Autodesk Inventor part; units mm, degrees
ref_plane "YZ Plane" through (0, 0, 0) normal (1, 0, 0) x (0, 1, 0)
ref_plane "XZ Plane" through (0, 0, 0) normal (0, 1, 0) x (-1, 0, 0)
ref_plane "XY Plane" through (0, 0, 0) normal (0, 0, 1) x (1, 0, 0)
sketch "Sketch1" plane through (0, 0, 0) normal (0, 1, 0) x (-1, 0, 0)
  line L0 (-25, 25) -> (25, 25)
  line L1 (25, 25) -> (25, -25)
  line L2 (25, -25) -> (-25, -25)
  line L3 (-25, -25) -> (-25, 25)
  line L4 (-25, 25) -> (25, -25) construction
  line L5 (25, 25) -> (-25, -25) construction
  line L6 (25, 0) -> (-25, 0)
  circle A0 centre (12.5, 15.25) radius 1.75
  line L7 (-25, 12.5) -> (0, 12.5)
  line L8 (-12.5, 12.5) -> (-12.5, 0)
  circle A1 centre (-12.5, 6.25) radius 1.75
  line L9 (25, -25) -> (-25, 25) construction
  circle A2 centre (12.5, -15.25) radius 1.75
  circle A3 centre (-12.5, -6.25) radius 1.75
  line L10 (0, 32.5) -> (50, 32.5)
  line L11 (50, 32.5) -> (50, -32.5)
  line L12 (50, -32.5) -> (0, -32.5)
  line L13 (0, -32.5) -> (0, 32.5)
  line L14 (0, 32.5) -> (50, -32.5) construction
  line L15 (50, 32.5) -> (0, -32.5) construction
  line L16 (50, -32.5) -> (29.5652, -32.5)
  line L17 (29.5652, -32.5) -> (29.5652, 32.5)
  line L18 (29.5652, 32.5) -> (50, 32.5)
  line L19 (0, 32.5205) -> (0, -32.5)
  circle A4 centre (12.5, -15.25) radius 15
  line L20 (29.5652, -32.5) -> (39.5652, -32.5)
  line L21 (39.5652, -32.5) -> (39.5652, 32.5)
  line L22 (39.5652, 32.5) -> (29.5652, 32.5)
  line L23 (29.5652, 32.5) -> (29.5652, -32.5)
  line L24 (12.5, -15.25) -> (12.5, 0)
  line L25 (-12.5, -6.25) -> (12.5, -6.25)
  circle A5 centre (-4, 0) radius 5
  circle A6 centre (-4, 0) radius 1.75
  line L26 (0, 0) -> (-4, 0)
  line L27 (29.5652, -32.5) -> (29.5652, -27.5)
  line L28 (29.5652, -27.5) -> (34.5652, -27.5)
  line L29 (34.5652, -27.5) -> (34.5652, 27.5)
  line L30 (34.5652, 27.5) -> (29.5652, 27.5)
  line L31 (29.5652, 27.5) -> (29.5652, -27.5)
  point P0 (0, -12.5)
  point P1 (-12.5, -12.5)
  point P2 (0, 25)
  point P3 (0, -25)
  point P4 (0, 25)
  point P5 (0, -25)
  point P6 (0, 32.5)
  point P7 (0, 32.5)
  point P8 (0, -23.5416)
  point P9 (1.101, -25)
  point P10 (25, -23.5416)
  point P11 (23.899, -25)
  point P12 (39.5652, 32.5)
  point P13 (0, 0)
  dimension "d0" = 50
  dimension "d1" = 50
  dimension "d5" = 3.5
  dimension "d7" = 3.5
  dimension "d11" = 15.25
  dimension "d12" = 50
  dimension "d13" = 65
  dimension "d19" = 30
  dimension "d21" = 10
  dimension "d27" = 7.5
  dimension "d28" = 7.5
  dimension "d31" = 9
  dimension "d32" = 25
  dimension "d57" = 10
  dimension "d58" = 3.5
  dimension "d59" = 4
  dimension "d60" = 5
  dimension "d61" = 55
extrude "Extrusion3" add sketch "Sketch1" along normal blind 5 contours L0 L13 L7 L3 | L13 L10 L17 L12 L2 A4 L1 L0 | L0 L1 L6 A5 L13 | L7 L8 A1 L6 L3 | L13 A5 L6 L8 A1 L7 | L6 A5 L13 A4 L2 L3 | L1 A4 L24 L6 | A5 L6 L13 | L13 L6 A6 A5 | A4 L1 | L1 A4 L2 L13 L25 L24 | L24 A4 L25 L13 A5 L6 | L13 A5 L6 A6 | L6 A5 L13 | L30 L29 L28 L17 | L13 A4 L2 | L1 L2 A4 | L24 L25 A4 | L2 A4 | A4 L13 | A4 L13 L25 | A0
fillet "Fillet5" radius 12 2 edges at (0, 2.5, 32.5) (0, 2.5, -32.5)
fillet "Fillet6" radius 12 2 edges at (0, 2.5, 25) (0, 2.5, -25)
fillet "Fillet7" radius 18.5 2 edges at (25, 2.5, 25) (25, 2.5, -25)
sketch "Sketch5" plane through (0, 5, 0) normal (0, 1, 0) x (1, 0, 0)
  circle A0 centre (-12.5, 15.25) radius 1.75
  circle A1 centre (-12.5, -15.25) radius 1.5
  circle A2 centre (-12.5, -15.25) radius 5
  circle A3 centre (4, 0) radius 1.75
  circle A4 centre (4, 0) radius 3
  circle A5 centre (12.5, 6.25) radius 1.75
  circle A6 centre (12.5, 6.25) radius 3
  circle A7 centre (12.5, -6.25) radius 1.75
  circle A8 centre (12.5, -6.25) radius 3
  circle A9 centre (-12.5, 15.25) radius 3
  point P0 (0, 0)
  dimension "d63" = 6
  dimension "d64" = 6
  dimension "d65" = 6
  dimension "d71" = 10
  dimension "d75" = 6
extrude "Extrusion8" cut sketch "Sketch5" against normal blind 2 contours A3 | A4 | A5 | A6 | A7 | A8
fillet "Fillet9" radius 2 11 edges at (6.4021, 5, 25) (1.5607, 5, 25.9773) (-6.3809, 5, 31.5227) (-20.3448, 5, 32.5) (25, 5, 0) (19.5815, 5, -19.5815) (6.4021, 5, -25) (1.5607, 5, -25.9773) (-6.3809, 5, -31.5227) (-20.3448, 5, -32.5) (19.5815, 5, 19.5815)
extrude "Extrusion9" cut sketch "Sketch5" against normal through all contours A1 | A2
sketch "Sketch6" plane through (0, 0, 0) normal (0, -1, 0) x (1, 0, 0)
  circle A0 centre (-12.5, -15.25) radius 1.75
  circle A1 centre (-12.5, -15.25) radius 5
  point P0 (0, 0)
  dimension "d72" = 10
extrude "Extrusion10" cut sketch "Sketch6" against normal blind 2
extrude "Extrusion11" cut sketch "Sketch5" against normal blind 2 contours A0 | A9
sketch "Sketch7" plane through (0, 0, 0) normal (0, -1, 0) x (1, 0, 0)
  circle A0 centre (-12.5, 15.25) radius 5
  circle A1 centre (-12.5, -15.25) radius 5
  point P0 (0, 0)
  point P1 (-12.5, 20.25)
  point P2 (-12.5, -20.25)
properties part number "Top"
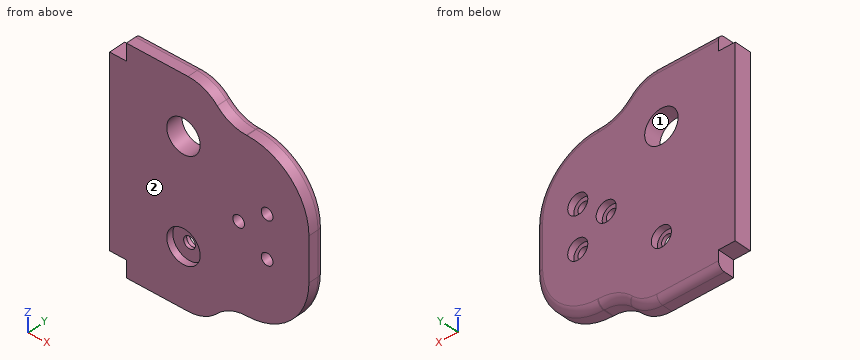
Check sheet for the modelled part. Datum: model origin and axes. Units: mm. Face numbers are marked on the shaded views. Give positions to 0.01 mm unless a question says otherwise; leave off trailing zeros. Write each loop counter-clockwise with the first axis right and the second up, starting at its lowest first coordinate (ties: lowest second). Pieces come first, ordered by that corner, then holes. Notation, with made-up numbers: (-16, -17.5) - (41, -17.5) arc R15 cw to (41, -7.5) - close; hole circle Ø10 at (-5.5, -39). An arc over 180 degrees is marked (long way). Answer as a JSON object with one key per item and string values. Group by question number.
1) Thickness scan on probe 1 along Z at (x, y) = (-12.5, 2.8); probe 2 along Z at (x, y) = (12.5, 3.65); probe 3 along X at (y, z) = (4.05, 0). Record the ranges inside material, lowest first. Write a range as from..to.
2) Release check for a two-part mould opening along Z. For the marked faces 1 and 2 record: pulls with the +Z half, pulls with the -Z half, needs draft (parallel to the pull), parting line crosses it, or undercut.
3) Depth check by flat-ended pin: P1, Ø5.5, axis at x = 4, z = 0, coming from the +Y side; P2, Ø2.5, axis at x = -31, y = 3, coming from the +Z side; P3, Ø1.5, axis at y = 3.5, z = -29, coming from the -X side; P4, Ø3, axis at x = 12.5, z = -6.25, coming from the +Y side. Enter the tip coordinate at first touch or a pass-through.
4) Sectioned sample at A-A (z = 0). Record the cut outline in (x, y).
5) Sectioned sample at B-B (x = -13.5). Record the cut outline in (y, z), then the cut area to 3 significant figures.
Geometry results:
{
 "1": {"probe 1": "z = -32.5..-17, -13.5..10.25, 20.25..32.5", "probe 2": "z = -23.89..-9.25, -3.25..3.25, 9.25..23.89", "probe 3": "x = -34.57..1, 7..24.7"},
 "2": {"face 1": "undercut", "face 2": "needs draft"},
 "3": {"P1": "stops at y = 3", "P2": "stops at z = 27.5", "P3": "stops at x = -29.57", "P4": "passes through"},
 "4": {"outline": "(-34.57, 0) - (2.25, 0) - (2.25, 3) - (1, 3) - (1, 5) - (-34.57, 5) - close; (5.75, 0) - (25, 0) - (25, 3) arc R2 ccw to (23, 5) - (7, 5) - (7, 3) - (5.75, 3) - close"},
 "5": {"outline": "(0, -32.5) - (3, -32.5) arc R2 ccw to (5, -30.5) - (5, -18.08) - (3, -18.08) - (3, -16.69) - (2, -16.69) - (2, -20.15) - (0, -20.15) - close; (0, -10.35) - (2, -10.35) - (2, -13.81) - (3, -13.81) - (3, -12.42) - (5, -12.42) - (5, 10.35) - (0, 10.35) - close; (0, 20.15) - (5, 20.15) - (5, 30.5) arc R2 ccw to (3, 32.5) - (0, 32.5) - close", "area": "241 mm^2"}
}
